from build123d import *

# Parameters (mm, degrees)
F0_W     = 150
F0_H     = 150
F0_W_2   = 35
F0_H_2   = 35
F1_DEPTH = 10
F2_DEPTH = 9.8


with BuildPart() as f1:
    # F0 (on Top) → F1 (new body)
    with BuildSketch(Plane.XY):
        Rectangle(F0_W, F0_H)
        with Locations((-45, -45)):
            Rectangle(F0_W_2, F0_H_2, mode=Mode.SUBTRACT)
        with Locations((0, -45)):
            Rectangle(F0_W_2, F0_H_2, mode=Mode.SUBTRACT)
        with Locations((45, -45)):
            Rectangle(F0_W_2, F0_H_2, mode=Mode.SUBTRACT)
        with Locations((-45, 0)):
            Rectangle(F0_W_2, F0_H_2, mode=Mode.SUBTRACT)
        with Locations((-45, 45)):
            Rectangle(F0_W_2, F0_H_2, mode=Mode.SUBTRACT)
        Rectangle(F0_W_2, F0_H_2, mode=Mode.SUBTRACT)
        with Locations((45, 0)):
            Rectangle(F0_W_2, F0_H_2, mode=Mode.SUBTRACT)
        with Locations((0, 45)):
            Rectangle(F0_W_2, F0_H_2, mode=Mode.SUBTRACT)
        with Locations((45, 45)):
            Rectangle(F0_W_2, F0_H_2, mode=Mode.SUBTRACT)
    extrude(amount=F1_DEPTH)

    # F0 (on Top) → F2 (join)
    with BuildSketch(Plane.XY):
        with Locations((-45, 45)):
            Rectangle(F0_W_2, F0_H_2)
        with Locations((-45, 0)):
            Rectangle(F0_W_2, F0_H_2)
        with Locations((-45, -45)):
            Rectangle(F0_W_2, F0_H_2)
        with Locations((0, -45)):
            Rectangle(F0_W_2, F0_H_2)
        Rectangle(F0_W_2, F0_H_2)
        with Locations((0, 45)):
            Rectangle(F0_W_2, F0_H_2)
        with Locations((45, 45)):
            Rectangle(F0_W_2, F0_H_2)
        with Locations((45, 0)):
            Rectangle(F0_W_2, F0_H_2)
        with Locations((45, -45)):
            Rectangle(F0_W_2, F0_H_2)
    extrude(amount=F2_DEPTH)


solid = f1.part
Here's how the part is built. I have some questions about the finished solid (model axes, mm). A direction names the side the tool comes from. Round coordinates to 2 decimals unless told otherwise and drop trailing zeros.
1. For P1, Ø10.5, axis at x = -49, y = -37.5, coming from the +Z side, with a flat end and sliding along its axis, tell me the tip position at first contact or that it passes through.
Answer list:
P1: stops at z = 9.8
2. If I drill on line 1 along Z through (x, y) = (28, -54.5), over which ranges is the centre line in solid material (lowest first)?
Answer list:
line 1: z = 0 to 9.8
3. We'd pull the mould along X, two halves only. Please class faces 1 (the face through (75, -1, 5)), 2 (the face through (-45, 0, 9.8)), 3 (the face through (-1, 18, 10)), 4 (the face through (-45, -45, 9.8)): +X half, -X half, draft (parallel to the pull), parting line (faces both ways), or undercut.
Answer list:
face 1: +X half
face 2: undercut
face 3: draft
face 4: undercut
4. Which directions (+Z, -Z, +X, -X, +Y, -Y) give clear straight access to the entire face, cutting with the end or side of a thin tool? Please do faces 5 (the face through (-1, -75, 5)), 6 (the face through (0, -45, 9.8)).
Answer list:
face 5: +Z, -Z, +X, -X, -Y
face 6: +Z
